```python
from build123d import *

# Parameters (mm, degrees)
F1_DEPTH = 6.35
F2_R     = 0.254
F3_R     = 0.508


with BuildPart() as f1:
    # F0 (on Front) → F1 (new body)
    with BuildSketch(Plane.XZ):
        with BuildLine():
            Line((4.466619, 2.85162), (0, 0))
            Line((0, 0), (6.35, 0))
            Line((6.35, 0), (6.35, 15.875))
            Line((6.35, 15.875), (1.905, 15.875))
            ThreePointArc((1.905, 15.875), (0.031846, 14.316871), (1.222856, 12.191319))
            ThreePointArc((1.222856, 12.191319), (1.672644, 11.664932), (1.476048, 11.001048))
            Line((1.476048, 11.001048), (0, 9.525))
            Line((0, 9.525), (1.779807, 9.369287))
            ThreePointArc((1.779807, 9.369287), (2.998749, 8.355504), (2.476049, 6.858721))
            Line((2.476049, 6.858721), (0, 5.059766))
            Line((0, 5.059766), (4.14303, 4.403575))
            ThreePointArc((4.14303, 4.403575), (4.840359, 3.739258), (4.466619, 2.85162))
        make_face()
    extrude(amount=F1_DEPTH)

    # F2
    f2_edges = [f1.edges().sort_by_distance(p)[0] for p in [
        (0, -3.175, 0),
        (0, -3.175, 9.525),
    ]]
    fillet(f2_edges, radius=F2_R)

    # F3
    f3_edges = [f1.edges().sort_by_distance(p)[0] for p in [
        (6.35, -3.175, 0),
        (6.35, -3.175, 15.875),
        (0, -3.175, 5.059766),
    ]]
    fillet(f3_edges, radius=F3_R)


solid = f1.part
```
Check sheet for the modelled part. Datum: model origin and axes. Units: mm. A direction names the side the tool comes from. Round coordinates to 2 decimals unless told otherwise and drop trailing zeros. Loops run counter-clockwise (first coordinate to the right, second up) from the corner with the lowest first, then second, coordinate; pieces in that order, holes last. Notation, with made-up numbers: (85.5, 35.5) - (106.5, 35.5) arc R19 cw to (106.5, 71.5) - close; hole circle Ø4 at (-37.5, 18). An arc over 180 degrees is marked (long way). Write item = value, one per line. Start each with the question number.
Q1. Section check A-A (y = -3.25). Record the boundary of the cut face in (x, z) (3 decimals), plus the area to 3 significant figures.
Q2. Access from +Z, -Z, +X, -X, +Y, -Y to the whole of each face (thin tool, end or side, straight path). Record for faces 1 (the face through (6.35, -3, 8)), 2 (the face through (1.745, -3.131, 6.327)).
Q3. Section check C-C (z = 14.75). Record the boundary of the cut face in (x, y).
Q4. Depth check by flat-ended pin: P1, Ø1.5, axis at y = -3.5, z = 12.5, coming from the -X side. Enter the tip coordinate at first touch or a pass-through.
Q5. Release check for a two-part mould opening along Z. For faces 3 (the face through (2.99, -3.13, 8.38)), 4 (the face through (4, 0, 8)), 5 (the face through (3, -3, 0)) record: pulls with the +Z half, pulls with the -Z half, needs draft (parallel to the pull), parting line crosses it, or undercut.
Q6. Thickness scan on L1, parallel to Z at x = 1, y = -3.25 (3 decimals); L2, parallel to Z at x = 0.75, y = -1.5 (3 decimals); L3, parallel to Z at x = 4, y = -5.25 (3 decimals). Record the ranges inside material, lowest first.
Q7. Section check B-B (x = 2.75). Record the boundary of the cut face in (y, z) (3 decimals), plus the area to 3 significant figures.
Q8. Section check D-D (z = 12.5). Record the boundary of the cut face in (x, y).
Derived:
q1.outline = (0.385, 9.91) arc R0.254 ccw to (0.543, 9.478) - (1.78, 9.369) arc R1.391 cw to (2.476, 6.859) - (0.992, 5.781) arc R0.508 ccw to (1.211, 4.868) - (4.143, 4.404) arc R0.848 cw to (4.467, 2.852) - (0.733, 0.468) arc R0.254 ccw to (0.87, 0) - (5.842, 0) arc R0.508 ccw to (6.35, 0.508) - (6.35, 15.367) arc R0.508 ccw to (5.842, 15.875) - (1.905, 15.875) arc R1.905 ccw to (1.223, 12.191) arc R0.725 cw to (1.476, 11.001) - close
q1.area = 71.4 mm^2
q2.face_1 = +Z, -Z, +X, +Y, -Y
q2.face_2 = -X, +Y, -Y
q3.outline = (0.17, -6.35) - (6.35, -6.35) - (6.35, 0) - (0.17, 0) - close
q4.P1 = 0.14
q5.face_3 = undercut
q5.face_4 = needs draft
q5.face_5 = pulls with the -Z half
q6.L1 = 0 to 0.638, 4.953 to 5.786, 9.438 to 10.525, 12.294 to 15.646
q6.L2 = 0.03 to 0.479, 9.459 to 10.275, 12.455 to 15.485
q6.L3 = 0 to 2.554, 4.426 to 15.875
q7.outline = (-6.35, 0) - (0, 0) - (0, 1.756) - (-6.35, 1.756) - close; (-6.35, 4.624) - (0, 4.624) - (0, 7.122) - (-6.35, 7.122) - close; (-6.35, 8.846) - (0, 8.846) - (0, 15.875) - (-6.35, 15.875) - close
q7.area = 71.6 mm^2
q8.outline = (0.69, -6.35) - (6.35, -6.35) - (6.35, 0) - (0.69, 0) - close
